```python
from build123d import *

# Parameters (mm, degrees)
BOSS_EXTRUDE1_DEPTH = 47.625
SKETCH2_R           = 6.35
BOSS_EXTRUDE2_DEPTH = 9.525
BOSS_EXTRUDE3_START = 9.525
SKETCH3_R           = 6.35
BOSS_EXTRUDE3_DEPTH = 9.525
CHAMFER2_SIZE       = 0.508


with BuildPart() as part:
    # Sketch1 → Boss-Extrude1 (new body)
    with BuildSketch(Plane(origin=(0, 0, 0), x_dir=(1, 0, 0), z_dir=(0, 1, 0))):
        Polygon((3.666174209, -6.35), (7.332348419, 0), (3.666174209, 6.35), (-3.666174209, 6.35), (-7.332348419, 0), (-3.666174209, -6.35), align=None)
    extrude(amount=BOSS_EXTRUDE1_DEPTH)

    # Sketch2 → Boss-Extrude2 (add)
    with BuildSketch(Plane(origin=(0, 0, 0), x_dir=(-1, 0, 0), z_dir=(0, -1, 0))):
        with Locations(Location((0, 0, 0), (0, 0, 90))):
            Circle(SKETCH2_R)
    extrude(amount=BOSS_EXTRUDE2_DEPTH)

    # Sketch3 → Boss-Extrude3 (add)
    with BuildSketch(Plane(origin=(0, 47.625, 0), x_dir=(1, 0, 0), z_dir=(0, 1, 0)).offset(BOSS_EXTRUDE3_START)):
        with Locations(Location((0, 0, 0), (0, 0, 90))):
            Circle(SKETCH3_R)
    extrude(amount=-BOSS_EXTRUDE3_DEPTH)

    # Chamfer2
    chamfer2_edges = [part.edges().sort_by_distance(p)[0] for p in [
        (0, -9.525, 6.35),
        (0, 57.15, 6.35),
    ]]
    chamfer(chamfer2_edges, length=CHAMFER2_SIZE)


solid = part.part
```
Check sheet for the modelled part. Datum: model origin and axes. Units: mm. A direction names the side the tool comes from. Coordinates: 2 decimals unless noted, no trailing zeros. Loops run counter-clockwise (first coordinate to the right, second up) from the corner with the lowest first, then second, coordinate; pieces in that order, holes last. Notation, with made-up numbers: M -22.5,11 L 2.5,11 A17 cw 2.5,25 Z; hole C -15.5,10 d2. An arc over 180 degrees is marked long. Answer as a JSON object with one key per item and string values.
1. Sectioned sample at A-A on y = 28.5. Record the cut outline in (x, z).
Outcome:
{"outline": "M -7.33,0 L -3.67,-6.35 L 3.67,-6.35 L 7.33,0 L 3.67,6.35 L -3.67,6.35 Z"}
2. Scan lines: L1, parallel to X at y = 29.5, z = -2.75; L2, parallel to X at y = 46.5, z = 4; L3, parallel to Z at x = -5, y = 53. Record each from-to range of solid material in increasing order. Write a range as from..to.
Outcome:
{"L1": "-5.74..5.74", "L2": "-5.02..5.02", "L3": "-3.91..3.91"}
3. Depth check by flat-ended pin: P1, Ø3, axis at y = 20.5, z = 4.5, coming from the -X side; P2, Ø0.9, axis at x = 6.5, z = 0, coming from the +Y side; P3, Ø0.5, axis at x = 6.5, z = 0.5, coming from the -Y side. Enter the tip coordinate at first touch or a pass-through.
Outcome:
{"P1": "x = -5.6", "P2": "y = 56.94", "P3": "y = -9.1"}
4. Access from +Z, -Z, +X, -X, +Y, -Y to the whole of each face (thin tool, end or side, straight path). Record for faces 1 (the cylindrical face through (-3.86, -4.45, 5.04)), 2 (the flat face through (3, 0, 6)), 3 (the flat face through (3, 47.625, 6)).
Outcome:
{"face 1": "-Y", "face 2": "+Z, +X, -Y", "face 3": "+Z, +X, +Y"}
5. Sectioned sample at B-B on y = -3.5. Record the cut outline in (x, z).
Outcome:
{"outline": "C 0,0 d12.7"}
